from build123d import *

# Parameters (mm, degrees)
SKETCH2_R           = 3.175
BOSS_EXTRUDE1_DEPTH = 34.798
SKETCH3_R           = 3.175
BOSS_EXTRUDE2_DEPTH = 34.798


with BuildPart() as part:
    # Sketch1 → Revolve1 (revolve)
    with BuildSketch(Plane.XY, mode=Mode.PRIVATE) as revolve1_sk:
        with BuildLine():
            Line((15, 33.02), (15, 292.38))
            ThreePointArc((15, 292.38), (18.521588729, 296.916296192), (19.685, 302.54))
            Line((19.685, 302.54), (22.225, 302.54))
            Line((22.225, 302.54), (22.225, 312.7))
            Line((22.225, 312.7), (3.175, 312.7))
            Line((3.175, 312.7), (3.175, 325.4))
            Line((3.175, 325.4), (0, 325.4))
            Line((0, 325.4), (0, 0))
            Line((0, 0), (3.175, 0))
            Line((3.175, 0), (3.175, 12.7))
            Line((3.175, 12.7), (22.225, 12.7))
            Line((22.225, 12.7), (22.225, 22.86))
            Line((22.225, 22.86), (19.685, 22.86))
            ThreePointArc((19.685, 22.86), (18.521588729, 28.483703808), (15, 33.02))
        make_face()
    revolve(revolve1_sk.sketch.rotate(Axis((0, -1025.4, 0), (0, 1, 0)), 90), axis=Axis((0, -1025.4, 0), (0, 1, 0)))

    # Sketch2 → Boss-Extrude1 (add)
    with BuildSketch(Plane(origin=(0, 0, 0), x_dir=(0, 0, -1), z_dir=(1, 0, 0))):
        with Locations(Location((0, 307.62, 0), (0, 0, 180))):
            Circle(SKETCH2_R)
    extrude(amount=BOSS_EXTRUDE1_DEPTH)

    # Sketch3 → Boss-Extrude2 (add)
    with BuildSketch(Plane.XY):
        with Locations((0, 17.78)):
            Circle(SKETCH3_R)
    extrude(amount=-BOSS_EXTRUDE2_DEPTH)


solid = part.part
The model under review builds one solid part; all positions refer to its coordinate system, in mm. A direction names the side the tool comes from. Round coordinates to 2 decimals unless told otherwise and drop trailing zeros. Order: outer loops, then holes, each group sorted by start corner. A loop starts at its lowest first (then second) coordinate and runs counter-clockwise, first axis right, second up. Notation, with made-up numbers: (82, 33.25) -> (88, 33.25) arc R24 ccw to (88, 46.25) -> close; hole circle Ø4 at (-32.5, -1.75). An arc over 180 degrees is marked (long way). Return JSON: item names as keys, results as strings.
1. For faces 1 (the face through (-0.69, 14.68, -28.31)), 2 (the face through (1.93, 6.44, 2.52)), 3 (the face through (20, 302.54, -2)), list the 3-axis set-ups (+Z, -Z, +X, -X, +Y, -Y) from which the entire face can be reached by the end or side of a thin tool; tool diameter is ignored.
Answer block:
{"face 1": "-Z", "face 2": "-Y", "face 3": "none"}
2. Take a section at C-C (y = 131.5). Write out the cut boundary in (x, z).
Answer block:
{"outline": "circle Ø30 at (0, 0)"}
3. The part is to be moulded in two halves that separate along Y. For faces 4 (the face through (5, 12.7, 0)), 5 (the face through (20, 22.86, 2)), 6 (the face through (5, 312.7, 0)), 7 (the face through (-12.65, 164.52, -8.06)), say which applies: +Y half, -Y half, draft (parallel to the pull), parting line (faces both ways), or undercut.
Answer block:
{"face 4": "-Y half", "face 5": "undercut", "face 6": "+Y half", "face 7": "undercut"}
4. Take a section at A-A (z = -29.5). Write out the cut boundary in (x, y) (3 decimals).
Answer block:
{"outline": "circle Ø6.35 at (0, 17.78)"}
5. Take a section at B-B (y = 307.62). Write out the cut boundary in (x, z) (3 decimals), then the cut area to 3 significant figures.
Answer block:
{"outline": "(21.997, -3.175) -> (34.798, -3.175) -> (34.798, 3.175) -> (21.997, 3.175) arc R22.225 ccw (long way) to start", "area": "1,630 mm²"}
6. For L1, parallel to Y at x = 5.5, z = 19; L2, parallel to Y at x = 10.5, z = -4; L3, parallel to X at y = 67.5, z = 0, list the stretches that pass through material, from the lowest coordinate up. Write a range as [from, to].
Answer block:
{"L1": "y = [12.7, 22.86], [302.54, 312.7]", "L2": "y = [12.7, 312.7]", "L3": "x = [-15, 15]"}
7. Insertion check: P1, Ø1.5, axis at x = -6, y = 161.5, coming from the +Z side; P2, Ø3, axis at x = 14.5, y = 261.5, coming from the -Z side; P3, Ø2, axis at x = -10.5, y = 146.5, coming from the -Z side. Each pin has a flat end and moves straight along its axis. Give the tip position at first contact, or say it passes through.
Answer block:
{"P1": "stops at z = 14.05", "P2": "stops at z = -7.48", "P3": "stops at z = -11.61"}
